from build123d import *

# Parameters (mm, degrees)
F1_DEPTH = 12.7
F2_SIZE  = 5.08
F4_DEPTH = 12.7
F5_SIZE  = 6.34999


# Not quite as in the source:
# - a fillet or chamfer is up to 0.001 mm smaller than in the source, because OpenCascade refuses the exact size


with BuildPart() as f1:
    # F0 (on Top) → F1 (new body)
    with BuildSketch(Plane.XY):
        with BuildLine():
            Line((0, 190.5), (0, 12.7))
            ThreePointArc((0, 12.7), (3.7197438789, 3.7197438789), (12.7, 0))
            Line((12.7, 0), (342.9, 0))
            ThreePointArc((342.9, 0), (351.8802561211, 3.7197438789), (355.6, 12.7))
            Line((355.6, 12.7), (355.6, 190.5))
            ThreePointArc((355.6, 190.5), (351.8802561211, 199.4802561211), (342.9, 203.2))
            Line((342.9, 203.2), (12.7, 203.2))
            ThreePointArc((12.7, 203.2), (3.7197438789, 199.4802561211), (0, 190.5))
        make_face()
    extrude(amount=F1_DEPTH)

    # F2
    f2_edges = [f1.edges().sort_by_distance(p)[0] for p in [
        (0, 101.6, 12.7),
    ]]
    chamfer(f2_edges, length=F2_SIZE)

    # F3 (on face) → F4 (join)
    with BuildSketch(Plane.XY.offset(12.7)):
        with BuildLine():
            Line((17.78, 179.07), (17.78, 101.6))
            Line((17.78, 101.6), (17.78, 24.13))
            ThreePointArc((17.78, 24.13), (19.6398719395, 19.6398719395), (24.13, 17.78))
            Line((24.13, 17.78), (177.8, 17.78))
            Line((177.8, 17.78), (331.47, 17.78))
            ThreePointArc((331.47, 17.78), (335.9601280605, 19.6398719395), (337.82, 24.13))
            Line((337.82, 24.13), (337.82, 101.6))
            Line((337.82, 101.6), (337.82, 179.07))
            ThreePointArc((337.82, 179.07), (335.9601280605, 183.5601280605), (331.47, 185.42))
            Line((331.47, 185.42), (177.8, 185.42))
            Line((177.8, 185.42), (24.13, 185.42))
            ThreePointArc((24.13, 185.42), (19.6398719395, 183.5601280605), (17.78, 179.07))
        make_face()
    extrude(amount=F4_DEPTH)

    # F5 (size 6.35 in the source; OpenCascade refuses exactly that, so slightly less here)
    f5_edges = [f1.edges().sort_by_distance(p)[0] for p in [
        (177.8, 17.78, 25.4),
    ]]
    chamfer(f5_edges, length=F5_SIZE)


solid = f1.part
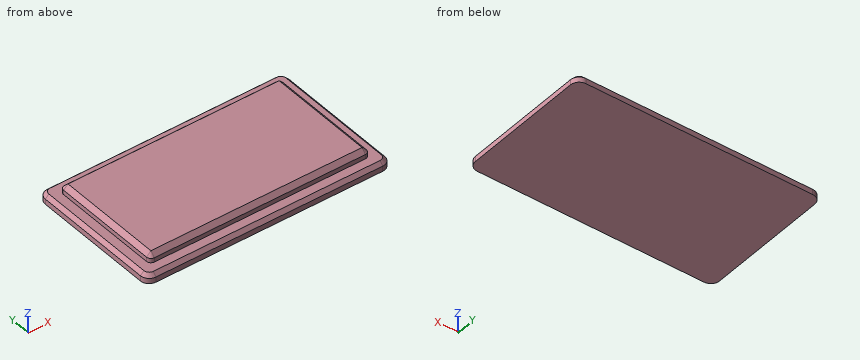
Here's how the part is built. I have some questions about the finished solid (model axes, mm). Coordinates: 2 decimals unless noted, no trailing zeros. Loops run counter-clockwise (first coordinate to the right, second up) from the corner with the lowest first, then second, coordinate; pieces in that order, holes last.
1. Imagine slicing it at A-A, the plane x = 217.5. Please give me the cut outline in (y, z), and give its area (3 significant figures).
2. Imagine slicing it at B-B, the plane y = 38.5. Please give me the cut outline in (x, z), and give its area (3 significant figures).
3. For P1, Ø10, axis at y = 40, z = 16, coming from the +X side; P2, Ø3, axis at x = 212.5, z = 17.5, coming from the +Y side; P3, Ø5, axis at y = 104, z = 15, coming from the -X side, each with a flat end and sliding along its axis, tell me the tip position at first contact or that it passes through.
4. I need wall thicknesses on L1, parallel to X at y = 64.5, z = 15.75; L2, parallel to Y at x = 30.5, z = 16.5; L3, parallel to Z at x = 37, y = 189.5. Which ranges of each line are inside material? Lowest first, please.
Taken from the geometry:
1. outline: (0, 0) - (203.2, 0) - (203.2, 7.62) - (198.12, 12.7) - (185.42, 12.7) - (185.42, 19.05) - (179.07, 25.4) - (24.13, 25.4) - (17.78, 19.05) - (17.78, 12.7) - (5.08, 12.7) - (0, 7.62) - close
1. area: 4,640 mm2
2. outline: (0, 0) - (355.6, 0) - (355.6, 7.62) - (350.52, 12.7) - (337.82, 12.7) - (337.82, 19.05) - (331.47, 25.4) - (24.13, 25.4) - (17.78, 19.05) - (17.78, 12.7) - (5.08, 12.7) - (0, 7.62) - close
2. area: 8,510 mm2
3. P1: stops at x = 352.22
3. P2: stops at y = 185.42
3. P3: stops at x = 4.88
4. L1: x = 17.78 to 337.82
4. L2: y = 17.78 to 185.42
4. L3: z = 0 to 12.7
